For this review, use the dimensioned drawing (mm, ordinates from the lowest corner) and the shaded views. Round coordinates to 2 decimals unless told otherwise and drop trailing zeros. Write each loop counter-clockwise with the first axis right and the second up, starting at its lowest first coordinate (ties: lowest second). Pieces come first, ordered by that corner, then holes. Notation, with made-up numbers: (80, 41) -> (127, 41) arc R27 ccw to (127, 61) -> close; hole circle Ø5 at (69.25, 53). An arc over 180 degrees is marked (long way). Write each question's results on one line, items separated by ' | '. Start each with the question number.
Item 1: Add section B-B (x = 20). State the section outline as (y, z) points.
Item 2: To check wall thickness, follow line 1 along X through (y, z) = (0.4, 3); line 2 along Z through (x, y) = (15.5, 0.4); line 3 along Y through (x, z) = (29, 11.25). State the ranges of each line that lie inside material, in increasing order.
Item 3: Add section A-A (z = 8). State the section outline as (x, y) points.
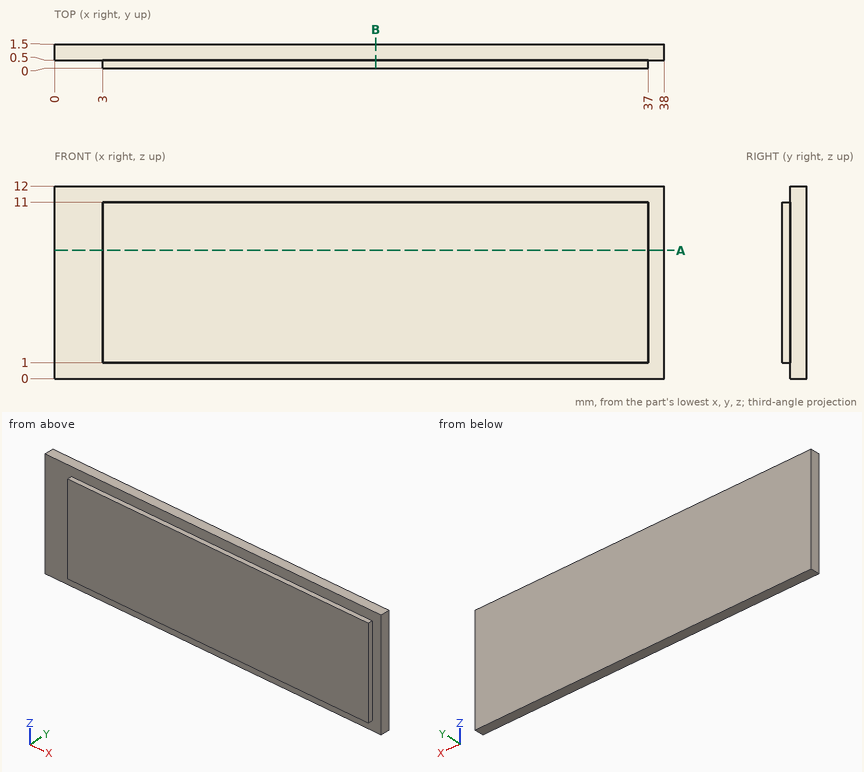
Responses:
1) outline: (0, 1) -> (0.5, 1) -> (0.5, 0) -> (1.5, 0) -> (1.5, 12) -> (0.5, 12) -> (0.5, 11) -> (0, 11) -> close
2) line 1: x = 3 to 37 | line 2: z = 1 to 11 | line 3: y = 0.5 to 1.5
3) outline: (0, 0.5) -> (3, 0.5) -> (3, 0) -> (37, 0) -> (37, 0.5) -> (38, 0.5) -> (38, 1.5) -> (0, 1.5) -> close
